Check sheet for the modelled part. Datum: model origin and axes. Units: mm. Face numbers are marked on the shaded views. A direction names the side the tool comes from. Give positions to 0.01 mm unless a question says otherwise; leave off trailing zeros. Order: outer loops, then holes, each group sorted by start corner. A loop starts at its lowest first (then second) coordinate and runs counter-clockwise, first axis right, second up. Notation, with made-up numbers: (-13, 61) - (10, 61) arc R22 ccw to (10, 100) - close; hole circle Ø9 at (-32, 55.5). An arc over 180 degrees is marked (long way). Answer in a Markdown table with one row per item.
Autodesk Inventor part; units mm, degrees
ref_plane "Work Plane1" through (-88, 0, 34.1) normal (0, 0, 1) x (1, 0, 0)
ref_plane "YZ Plane" through (0, 0, 0) normal (1, 0, 0) x (0, 1, 0)
ref_plane "XZ Plane" through (0, 0, 0) normal (0, 1, 0) x (-1, 0, 0)
sketch "Sketch1" plane through (0, 0, 0) normal (0, 1, 0) x (-1, 0, 0)
  line L0 (0, 0) -> (0, 68.2)
  line L1 (0, 68.2) -> (10.6066, 78.8066)
  line L2 (10.6066, 78.8066) -> (68.3066, 78.8066)
  line L3 (68.3066, 78.8066) -> (74.5, 85)
  line L4 (74.5, 85) -> (88, 85)
  line L5 (0, 34.1) -> (80, 34.1) construction
  line L6 (0, 0) -> (10.6066, -10.6066)
  line L7 (10.6066, -10.6066) -> (68.3066, -10.6066)
  line L8 (68.3066, -10.6066) -> (74.5, -16.8)
  line L9 (74.5, -16.8) -> (88, -16.8)
  line L10 (88, 88.5) -> (73.0503, 88.5)
  line L11 (73.0503, 88.5) -> (66.8569, 82.3066)
  line L12 (66.8569, 82.3066) -> (9.1569, 82.3066)
  line L13 (9.1569, 82.3066) -> (-3.5, 69.6497)
  line L14 (-3.5, 69.6497) -> (-3.5, -1.4497)
  line L15 (-3.5, -1.4497) -> (9.1569, -14.1066)
  line L16 (9.1569, -14.1066) -> (66.8569, -14.1066)
  line L17 (66.8569, -14.1066) -> (73.0503, -20.3)
  line L18 (73.0503, -20.3) -> (88, -20.3)
  line L19 (88, 88.5) -> (88, 85)
  line L20 (88, -16.8) -> (88, -20.3)
  dimension "d0" = 68.2
  dimension "d1" = 15
  dimension "d2" = 135
  dimension "d5" = 135
  dimension "d6" = 88
  dimension "d7" = 3.5
  dimension "d18" = 13.5
  dimension "d19" = 50.9
extrude "Extrusion1" add sketch "Sketch1" along normal blind 85
sketch "Sketch2" plane through (3.5, 0, 69.6497) normal (0.7071068, 0, 0.7071068) x (0.7071068, 0, -0.7071068)
  line L0 (-17.8995, 0) -> (0, 0)
  line L1 (0, 0) -> (0, 85)
  line L2 (-17.8995, 85) -> (0, 85)
  line L3 (-17.8995, 0) -> (-17.8995, 85)
  line L4 (-1.4497, 85) -> (-16.4497, 85) construction
  line L5 (-8.9497, 85) -> (-8.9497, 0) construction
  line L6 (-17.8995, 0) -> (0, 0) construction
  circle A0 centre (-8.9497, 70) radius 2.6
  circle A1 centre (-8.9497, 15) radius 2.6
  point P0 (46.7749, 0)
  dimension "d10" = 5.2
  dimension "d11" = 5.2
  dimension "d12" = 15
  dimension "d13" = 15
extrude "Extrusion2" cut sketch "Sketch2" against normal up to next contours A0 | A1
ref_plane "Work Plane1" through (-88, 0, 34.1) normal (0, 0, 1) x (1, 0, 0)
mirror "Mirror1" about plane through (-88, 0, 34.1) normal (0, 0, 1) of "Extrusion2"
sketch "Sketch4" plane through (-10.6066, 0, 78.8066) normal (0, 0, -1) x (-1, 0, 0)
  line L0 (27.7, 12) -> (42.7, 12)
  line L1 (42.7, 12) -> (42.7, 0)
  line L2 (42.7, 0) -> (27.7, 0)
  line L3 (27.7, 0) -> (27.7, 12)
  line L4 (0, 85) -> (57.7, 85)
  line L5 (57.7, 0) -> (57.7, 85)
  line L6 (0, 0) -> (57.7, 0)
  point P0 (-10.6066, 0)
  dimension "d20" = 15
  dimension "d21" = 12
  dimension "d22" = 15
extrude "Extrusion4" add sketch "Sketch4" along normal blind 6
sketch "Sketch5" plane through (-53.3066, 0, 78.8066) normal (-1, 0, 0) x (0, 0, 1)
  line L0 (0, 12) -> (0, 0)
  line L1 (0, 12) -> (-6, 12)
  line L2 (-6, 0) -> (-6, 12)
  line L3 (0, 0) -> (-6, 0)
  line L4 (-3.75, 7) -> (-2.25, 7)
  line L5 (-2.25, 7) -> (-2.25, 5)
  line L6 (-2.25, 5) -> (-3.75, 5)
  line L7 (-3.75, 5) -> (-3.75, 7)
  line L8 (-6, 0) -> (-6, 12) construction
  line L9 (-6, 6) -> (-3.75, 6) construction
  line L10 (0, 12) -> (-6, 12) construction
  line L11 (-3, 12) -> (-3, 7) construction
  point P0 (-78.8066, 0)
  dimension "d25" = 1.5
  dimension "d26" = 2
extrude "Extrusion5" cut sketch "Sketch5" against normal up to next contours L4 L5 L6 L7
chamfer "Chamfer1" distance 3 distance2 6 1 edges at (-53.3066, 6, 72.8066) measured on face at (-43.3066, 8, 72.8066)
chamfer "Chamfer2" distance 3 distance2 6 1 edges at (-38.3066, 6, 72.8066) measured on face at (-42.3066, 8, 72.8066)
fillet "Fillet1" radius 6 2 edges at (-45.8066, 12, 72.8066) (-45.8066, 0, 72.8066)
equation "\"d11\" = d10"
equation "\"d13\" = d12"
properties part number "Z Axis Cover Bottom"
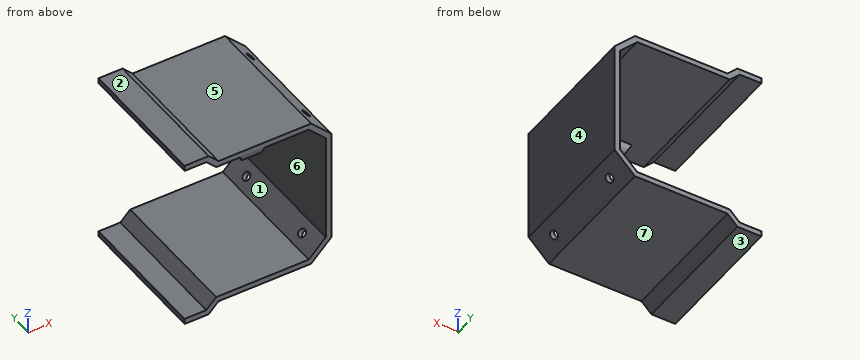
(1) Cross-section at A-A, the plane x = -48.5. Give the number of separate pieces and of enclosed holes in the cut face, then the cut area to 3 significant figures.
Geometry says:
| item | result |
|---|---|
| separate pieces | 2 |
| enclosed holes | 1 |
| area | 649 mm² |
(2) Access from +Z, -Z, +X, -X, +Y, -Y to the whole of each face (thin tool, end or side, straight path). Record for the marked faces 4, 5, 6 and 7.
Geometry says:
| item | result |
|---|---|
| face 4 | +Z, -Z, +X, +Y, -Y |
| face 5 | +Z, +X, +Y, -Y |
| face 6 | -X, +Y, -Y |
| face 7 | -Z, +X, +Y, -Y |
(3) Cross-section at D-D, the plane z = 15.5. Record the cut outline in (x, y).
Geometry says:
| item | result |
|---|---|
| outline | (0, 0) - (3.5, 0) - (3.5, 85) - (0, 85) - close |
(4) Thickness scan on L1, parallel to Z at x = -79, y = 27.5; L2, parallel to Z at x = -27.5, y = 42; L3, parallel to X at y = 13.5, z = 16. Record the ranges inside material, lowest first.
Geometry says:
| item | result |
|---|---|
| L1 | -20.3 to -16.8, 85 to 88.5 |
| L2 | -14.11 to -10.61, 78.81 to 82.31 |
| L3 | 0 to 3.5 |
(5) Cross-section at B-B, the plane x = -28. Record the cut outline in (y, z), then the cut area to 3 significant figures.
Geometry says:
| item | result |
|---|---|
| outline | (0, -14.11) - (85, -14.11) - (85, -10.61) - (0, -10.61) - close; (0, 78.81) - (85, 78.81) - (85, 82.31) - (0, 82.31) - close |
| area | 595 mm² |
(6) Gauge pin test, flat ends, axial feed: P1, Ø2, axis at x = -48, y = 6, coming from the +Z side; P2, Ø1.5, axis at y = 36, z = 70, coming from the -X side; P3, Ø6, axis at y = 53, z = 44.5, coming from the -X side. Record the tip position at first contact, or that the pin passes through.
Geometry says:
| item | result |
|---|---|
| P1 | z = 82.31 |
| P2 | x = -2.55 |
| P3 | x = 0 |
(7) Cross-section at C-C, the plane y = 64.5. Record the cut outline in (x, z), then the cut area to 3 significant figures.
Geometry says:
| item | result |
|---|---|
| outline | (-88, -20.3) - (-73.05, -20.3) - (-66.86, -14.11) - (-9.16, -14.11) - (3.5, -1.45) - (3.5, 69.65) - (-9.16, 82.31) - (-66.86, 82.31) - (-73.05, 88.5) - (-88, 88.5) - (-88, 85) - (-74.5, 85) - (-68.31, 78.81) - (-10.61, 78.81) - (0, 68.2) - (0, 0) - (-10.61, -10.61) - (-68.31, -10.61) - (-74.5, -16.8) - (-88, -16.8) - close |
| area | 924 mm² |
(8) Mould release check, pull along Z, two halves, no side actions. Record for the marked faces 1, 2 and 3: pulls with the +Z half, pulls with the -Z half, needs draft (parallel to the pull), parting line crosses it, or undercut.
Geometry says:
| item | result |
|---|---|
| face 1 | undercut |
| face 2 | pulls with the +Z half |
| face 3 | pulls with the -Z half |
